Geometry check sheet. Reference: the model listing, model coordinates, mm. Face numbers are marked on the shaded views. A direction names the side the tool comes from. Round coordinates to 2 decimals unless told otherwise and drop trailing zeros. Write each loop counter-clockwise with the first axis right and the second up, starting at its lowest first coordinate (ties: lowest second). Pieces come first, ordered by that corner, then holes. Notation, with made-up numbers: M 40.25,-32.75 L 75.25,-32.75 A26 ccw 75.25,-10.75 Z; hole C 18.5,-14.75 d7. An arc over 180 degrees is marked long. Answer as CSV lines item,"result". Start each with the question number.
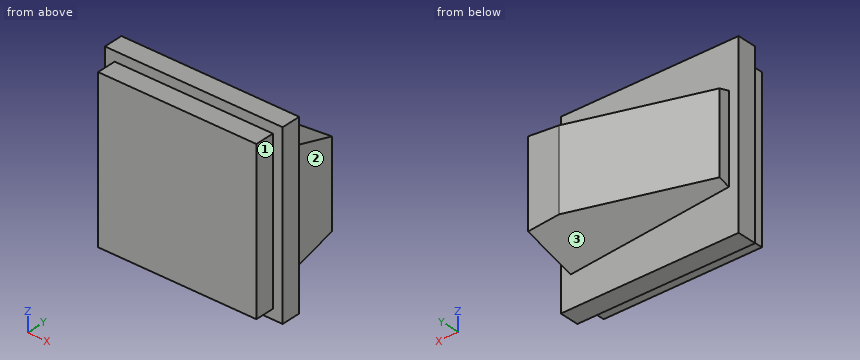
```python
from build123d import *

# Parameters (mm, degrees)
SKETCH2_W           = 812.8
SKETCH2_H           = 812.8
BOSS_EXTRUDE1_DEPTH = 457.2
SKETCH3_W           = 912.8
SKETCH3_H           = 912.8
SKETCH3_W_2         = 812.8
SKETCH3_H_2         = 812.8
BOSS_EXTRUDE2_DEPTH = 100
CHAMFER4_SIZE       = 200
CHAMFER4_SIZE2      = 654.170523697
CHAMFER5_SIZE       = 200
CHAMFER5_SIZE_2     = 654.170523697


with BuildPart() as part:
    # Sketch2 → Boss-Extrude1 (new body)
    with BuildSketch(Plane(origin=(0, 0, 0), x_dir=(1, 0, 0), z_dir=(0, 1, 0))):
        with Locations((406.4, 406.4)):
            Rectangle(SKETCH2_W, SKETCH2_H)
    extrude(amount=BOSS_EXTRUDE1_DEPTH)

    # Sketch3 → Boss-Extrude2 (add)
    with BuildSketch(Plane(origin=(0, 100, 0), x_dir=(1, 0, 0), z_dir=(0, 1, 0))):
        with Locations((406.4, 406.4)):
            Rectangle(SKETCH3_W, SKETCH3_H)
        with Locations((406.4, 406.4)):
            Rectangle(SKETCH3_W_2, SKETCH3_H_2, mode=Mode.SUBTRACT)
    extrude(amount=BOSS_EXTRUDE2_DEPTH)

    # Chamfer4
    chamfer4_edges = [part.edges().sort_by_distance(p)[0] for p in [
        (0, 457.2, -406.4),
    ]]
    chamfer4_side = [part.faces().sort_by_distance(p)[0] for p in [
        (0, 328.6, -406.4),
    ]]
    chamfer(chamfer4_edges, length=CHAMFER4_SIZE, length2=CHAMFER4_SIZE2, reference=chamfer4_side[0])

    # Chamfer5
    # the kernel refuses this chamfer: 654.170523697, 200 mm, written as the material it takes off along each edge
    with BuildSketch(Plane(origin=(-1623.89408898, -239.27424644, -812.8), x_dir=(-0.03497993633861633, 0.11441421636757278, 0.9928170985366542), z_dir=(0.9563047559630362, 0.2923717047227344, 0))) as chamfer5_piece_1_section:
        Polygon((CHAMFER5_SIZE * 0.992817098537, CHAMFER5_SIZE * 0.119642002881), (-CHAMFER5_SIZE_2 * 0.11964200288, CHAMFER5_SIZE_2 * 0.992817098536), (0, 0), align=None)
    chamfer5_piece_1 = extrude(amount=4080.246048475, mode=Mode.PRIVATE)
    chamfer5_piece_1 = split(chamfer5_piece_1, bisect_by=Plane(origin=(478.445479778, 200, -727.207473948), z_dir=(0, 1, 0)), keep=Keep.TOP, mode=Mode.PRIVATE)
    add(chamfer5_piece_1, mode=Mode.SUBTRACT)
    with BuildSketch(Plane(origin=(-1623.89408898, -239.27424644, 0), x_dir=(0.2923531587775955, -0.9562440949098164, 0.011263281176818211), z_dir=(0.9563047559630362, 0.2923717047227344, 0))) as chamfer5_piece_2_section:
        Polygon((CHAMFER5_SIZE_2 * 0.999936567236, CHAMFER5_SIZE_2 * 0.0112632811768), (-CHAMFER5_SIZE * 0.0112632811768, CHAMFER5_SIZE * 0.999936567237), (0, 0), align=None)
    chamfer5_piece_2 = extrude(amount=4080.246048475, mode=Mode.PRIVATE)
    chamfer5_piece_2 = split(chamfer5_piece_2, bisect_by=Plane(origin=(478.445479778, 200, -85.592526052), z_dir=(0, 1, 0)), keep=Keep.TOP, mode=Mode.PRIVATE)
    add(chamfer5_piece_2, mode=Mode.SUBTRACT)


solid = part.part
```
1) Section check D-D, the plane y = 351. Record the cut outline in (x, z), plus the area to 3 significant figures.
2) Access from +Z, -Z, +X, -X, +Y, -Y to the whole of each face (thin tool, end or side, straight path). Record for the marked faces 1, 2 and 3.
3) Section check C-C, the plane z = -747. Record the cut outline in (x, y).
4) Scan lines: line 1 (Y direction, x = 643.5, z = -707.5); line 2 (X direction, y = 52, z = -630); line 3 (Y direction, x = 818, z = -454.5). Record each from-to range of solid material in increasing order. Write a range as from..to.
5) Section check A-A, the plane z = -479. Record the cut outline in (x, y), plus the area to 3 significant figures.
6) Go/stop test with flat-tipped pins: pin 1 (8 mm diameter, centred on x = 362, y = 213, fed in from +Z); pin 2 (1.5 mm diameter, centred on y = 246, z = -608.5, fed in from +X); pin 3 (1.5 mm diameter, centred on x = 654.5, y = 364.5, fed in from -Z). Record where each tip stops, or that it passes through.
7) Section check B-B, the plane x = 677. Record the cut outline in (y, z).
Results:
1,outline,"M 306.81,-612.8 L 812.8,-658.03 L 812.8,-154.77 L 306.81,-200 Z"
1,area,"232,000 mm^2"
2,face 1,"+Z, -Z, +X, -Y"
2,face 2,"+Z, -Z, +X, +Y"
2,face 3,"-Z, -X, +Y"
3,outline,"M -50,100 L 0,100 L 0,0 L 812.8,0 L 812.8,100 L 862.8,100 L 862.8,200 L -50,200 Z"
4,line 1,"y = 0..200"
4,line 2,"x = 0..812.8"
4,line 3,"y = 100..200"
5,outline,"M -50,100 L 0,100 L 0,0 L 812.8,0 L 812.8,100 L 862.8,100 L 862.8,200 L 812.8,200 L 812.8,457.2 L 654.17,457.2 L 0,257.2 L 0,200 L -50,200 Z"
5,area,"316,000 mm^2"
6,pin 1,"stops at z = -153.5"
6,pin 2,"stops at x = 812.8"
6,pin 3,"stops at z = -640.16"
7,outline,"M 0,-812.8 L 100,-812.8 L 100,-862.8 L 200,-862.8 L 200,-690.04 L 457.2,-614.84 L 457.2,-197.96 L 200,-122.76 L 200,50 L 100,50 L 100,0 L 0,0 Z"
